Can you work these out from the model? Positions are in its coordinate system, mm. A direction names the side the tool comes from. Coordinates: 2 decimals unless noted, no trailing zeros. Order: outer loops, then holes, each group sorted by start corner. A loop starts at its lowest first (then second) coordinate and runs counter-clockwise, first axis right, second up. Notation, with made-up numbers: (-38.5, 0.5) -> (-8.5, 0.5) arc R35 cw to (-8.5, 36.5) -> close; hole circle Ø11 at (-13.5, -11.75). An arc over 180 degrees is marked (long way). Write item = value, one per line.
```python
from build123d import *
from OCP.BRepFilletAPI import BRepFilletAPI_MakeChamfer

# Parameters (mm, degrees)
SKETCH2_W           = 25.25
SKETCH2_H           = 38.25
SKETCH2_R           = 1.5
SKETCH2_W_2         = 19
SKETCH2_H_2         = 28.5
SKETCH2_R_2         = 1
BOSS_EXTRUDE1_DEPTH = 3
CHAMFER1_SIZE       = 0.5
CHAMFER1_SIZE2      = 0.360555128
CHAMFER1_SIZE2_2    = 0.382352941
CUT_EXTRUDE1_DEPTH  = 2
SKETCH5_R           = 1.5
SKETCH5_W           = 21
SKETCH5_H           = 28.5
BOSS_EXTRUDE2_DEPTH = 2.5


with BuildPart() as part:
    # Sketch2 → Boss-Extrude1 (new body)
    with BuildSketch(Plane.XY):
        Rectangle(SKETCH2_W, SKETCH2_H)
        with Locations((-10, -16.5)):
            Circle(SKETCH2_R, mode=Mode.SUBTRACT)
        with Locations((10, -16.5)):
            Circle(SKETCH2_R, mode=Mode.SUBTRACT)
        with Locations((10, 16.5)):
            Circle(SKETCH2_R, mode=Mode.SUBTRACT)
        with Locations((-10, 16.5)):
            Circle(SKETCH2_R, mode=Mode.SUBTRACT)
        Rectangle(SKETCH2_W_2, SKETCH2_H_2, mode=Mode.SUBTRACT)
        Polygon((-1.666666667, -1), (-1, 0), (-1.666666667, 1), (-9.5, 1), (-9.5, -1), align=None)
        with BuildLine():
            Line((-9.5, -14.25), (-8.833333333, -14.25))
            Line((-8.833333333, -14.25), (0, -1))
            ThreePointArc((0, -1), (-0.707106781, -0.707106781), (-1, 0))
            Line((-1, 0), (-1.666666667, -1))
            Line((-1.666666667, -1), (-9.5, -12.75))
            Line((-9.5, -12.75), (-9.5, -14.25))
        make_face()
        with BuildLine():
            Line((8.833333333, -14.25), (9.5, -14.25))
            Line((9.5, -14.25), (9.5, -12.75))
            Line((9.5, -12.75), (1.666666667, -1))
            Line((1.666666667, -1), (1, 0))
            ThreePointArc((1, 0), (0.707106781, -0.707106781), (0, -1))
            Line((0, -1), (8.833333333, -14.25))
        make_face()
        Polygon((1.666666667, -1), (9.5, -1), (9.5, 1), (1.666666667, 1), (1, 0), align=None)
        with BuildLine():
            ThreePointArc((0, 1), (0.707106781, 0.707106781), (1, 0))
            Line((1, 0), (1.666666667, 1))
            Line((1.666666667, 1), (9.5, 12.75))
            Line((9.5, 12.75), (9.5, 14.25))
            Line((9.5, 14.25), (8.833333333, 14.25))
            Line((8.833333333, 14.25), (0, 1))
        make_face()
        Circle(SKETCH2_R_2)
        with BuildLine():
            Line((-1.666666667, 1), (-1, 0))
            ThreePointArc((-1, 0), (-0.707106781, 0.707106781), (0, 1))
            Line((0, 1), (-8.833333333, 14.25))
            Line((-8.833333333, 14.25), (-9.5, 14.25))
            Line((-9.5, 14.25), (-9.5, 12.75))
            Line((-9.5, 12.75), (-1.666666667, 1))
        make_face()
    extrude(amount=BOSS_EXTRUDE1_DEPTH)

    # Chamfer1: one chamfer whose edges measure the first distance from different faces: ONE call of the kernel's chamfer builder (chamfer() names one face for all edges)
    chamfer1_edges_1 = [part.edges().sort_by_distance(p)[0] for p in [
        (-12.625, 19.125, 1.5),
        (12.625, 19.125, 1.5),
        (12.625, -19.125, 1.5),
        (-12.625, -19.125, 1.5),
        (-9.5, 1, 1.5),
        (-9.5, -1, 1.5),
        (9.5, -1, 1.5),
        (9.5, 1, 1.5),
    ]]
    chamfer1_edges_2 = [part.edges().sort_by_distance(p)[0] for p in [
        (-1.666666667, 1, 1.5),
    ]]
    chamfer1_side_2 = [part.faces().sort_by_distance(p)[0] for p in [
        (-5.583333333, 6.875, 1.5),
    ]]
    chamfer1_edges_3 = [part.edges().sort_by_distance(p)[0] for p in [
        (-9.5, 12.75, 1.5),
    ]]
    chamfer1_side_3 = [part.faces().sort_by_distance(p)[0] for p in [
        (-9.5, 6.875, 1.5),
    ]]
    chamfer1_edges_4 = [part.edges().sort_by_distance(p)[0] for p in [
        (-1.666666667, -1, 1.5),
    ]]
    chamfer1_side_4 = [part.faces().sort_by_distance(p)[0] for p in [
        (-5.583333333, -1, 1.5),
    ]]
    chamfer1_edges_5 = [part.edges().sort_by_distance(p)[0] for p in [
        (-9.5, -12.75, 1.5),
    ]]
    chamfer1_side_5 = [part.faces().sort_by_distance(p)[0] for p in [
        (-5.583333333, -6.875, 1.5),
    ]]
    chamfer1_edges_6 = [part.edges().sort_by_distance(p)[0] for p in [
        (8.833333333, 14.25, 1.5),
    ]]
    chamfer1_side_6 = [part.faces().sort_by_distance(p)[0] for p in [
        (0, 14.25, 1.5),
    ]]
    chamfer1_edges_7 = [part.edges().sort_by_distance(p)[0] for p in [
        (-8.833333333, 14.25, 1.5),
    ]]
    chamfer1_side_7 = [part.faces().sort_by_distance(p)[0] for p in [
        (-4.416666667, 7.625, 1.5),
    ]]
    chamfer1_edges_8 = [part.edges().sort_by_distance(p)[0] for p in [
        (0, 1, 1.5),
    ]]
    chamfer1_side_8 = [part.faces().sort_by_distance(p)[0] for p in [
        (4.416666667, 7.625, 1.5),
    ]]
    chamfer1_edges_9 = [part.edges().sort_by_distance(p)[0] for p in [
        (9.5, -12.75, 1.5),
    ]]
    chamfer1_side_9 = [part.faces().sort_by_distance(p)[0] for p in [
        (9.5, -6.875, 1.5),
    ]]
    chamfer1_edges_10 = [part.edges().sort_by_distance(p)[0] for p in [
        (1.666666667, -1, 1.5),
    ]]
    chamfer1_side_10 = [part.faces().sort_by_distance(p)[0] for p in [
        (5.583333333, -6.875, 1.5),
    ]]
    chamfer1_edges_11 = [part.edges().sort_by_distance(p)[0] for p in [
        (-8.833333333, -14.25, 1.5),
    ]]
    chamfer1_side_11 = [part.faces().sort_by_distance(p)[0] for p in [
        (0, -14.25, 1.5),
    ]]
    chamfer1_edges_12 = [part.edges().sort_by_distance(p)[0] for p in [
        (8.833333333, -14.25, 1.5),
    ]]
    chamfer1_side_12 = [part.faces().sort_by_distance(p)[0] for p in [
        (4.416666667, -7.625, 1.5),
    ]]
    chamfer1_edges_13 = [part.edges().sort_by_distance(p)[0] for p in [
        (0, -1, 1.5),
    ]]
    chamfer1_side_13 = [part.faces().sort_by_distance(p)[0] for p in [
        (-4.416666667, -7.625, 1.5),
    ]]
    chamfer1_edges_14 = [part.edges().sort_by_distance(p)[0] for p in [
        (9.5, 12.75, 1.5),
    ]]
    chamfer1_side_14 = [part.faces().sort_by_distance(p)[0] for p in [
        (5.583333333, 6.875, 1.5),
    ]]
    chamfer1 = BRepFilletAPI_MakeChamfer(part.part.solid().wrapped)
    for e in chamfer1_edges_1:
        chamfer1.Add(CHAMFER1_SIZE, e.wrapped)
    for e in chamfer1_edges_2:
        chamfer1.Add(CHAMFER1_SIZE, CHAMFER1_SIZE2, e.wrapped, chamfer1_side_2[0].wrapped)  # the first distance lies on this face
    for e in chamfer1_edges_3:
        chamfer1.Add(CHAMFER1_SIZE, CHAMFER1_SIZE2, e.wrapped, chamfer1_side_3[0].wrapped)  # the first distance lies on this face
    for e in chamfer1_edges_4:
        chamfer1.Add(CHAMFER1_SIZE, CHAMFER1_SIZE2, e.wrapped, chamfer1_side_4[0].wrapped)  # the first distance lies on this face
    for e in chamfer1_edges_5:
        chamfer1.Add(CHAMFER1_SIZE, CHAMFER1_SIZE2, e.wrapped, chamfer1_side_5[0].wrapped)  # the first distance lies on this face
    for e in chamfer1_edges_6:
        chamfer1.Add(CHAMFER1_SIZE, CHAMFER1_SIZE2, e.wrapped, chamfer1_side_6[0].wrapped)  # the first distance lies on this face
    for e in chamfer1_edges_7:
        chamfer1.Add(CHAMFER1_SIZE, CHAMFER1_SIZE2, e.wrapped, chamfer1_side_7[0].wrapped)  # the first distance lies on this face
    for e in chamfer1_edges_8:
        chamfer1.Add(CHAMFER1_SIZE, CHAMFER1_SIZE2_2, e.wrapped, chamfer1_side_8[0].wrapped)  # the first distance lies on this face
    for e in chamfer1_edges_9:
        chamfer1.Add(CHAMFER1_SIZE, CHAMFER1_SIZE2, e.wrapped, chamfer1_side_9[0].wrapped)  # the first distance lies on this face
    for e in chamfer1_edges_10:
        chamfer1.Add(CHAMFER1_SIZE, CHAMFER1_SIZE2, e.wrapped, chamfer1_side_10[0].wrapped)  # the first distance lies on this face
    for e in chamfer1_edges_11:
        chamfer1.Add(CHAMFER1_SIZE, CHAMFER1_SIZE2, e.wrapped, chamfer1_side_11[0].wrapped)  # the first distance lies on this face
    for e in chamfer1_edges_12:
        chamfer1.Add(CHAMFER1_SIZE, CHAMFER1_SIZE2, e.wrapped, chamfer1_side_12[0].wrapped)  # the first distance lies on this face
    for e in chamfer1_edges_13:
        chamfer1.Add(CHAMFER1_SIZE, CHAMFER1_SIZE2_2, e.wrapped, chamfer1_side_13[0].wrapped)  # the first distance lies on this face
    for e in chamfer1_edges_14:
        chamfer1.Add(CHAMFER1_SIZE, CHAMFER1_SIZE2, e.wrapped, chamfer1_side_14[0].wrapped)  # the first distance lies on this face
    add(Compound.cast(chamfer1.Shape()), mode=Mode.REPLACE)

    # Sketch3 → Cut-Extrude1 (cut)
    with BuildSketch(Plane(origin=(0, 0, 0), x_dir=(-1, 0, 0), z_dir=(0, 0, -1))):
        Polygon((10.5, -14.25), (10.5, 14.25), (8.472778206, 14.25), (8.555983235, 13.833974853), (0.212091251, 1.318136877), (-0.277350098, 1.416025147), (-8.633333333, 13.95), (-8.333333333, 14.25), (-10.5, 14.25), (-10.5, -14.25), (-8.472778206, -14.25), (-8.555983235, -13.833974853), (-0.212091251, -1.318136877), (0.277350098, -1.416025147), (8.633333333, -13.95), (8.333333333, -14.25), align=None)
        Polygon((-1.666666667, 1), (-9, 1), (-9.5, 1.5), (-9.5, 12.389444872), (-9.222649902, 12.333974853), align=None, mode=Mode.SUBTRACT)
        Polygon((-9.5, -1.5), (-9, -1), (-2.027221794, -1), (-1.944016765, -1.416025147), (-9.3, -12.45), (-9.5, -12.25), align=None, mode=Mode.SUBTRACT)
        Polygon((9.5, 1.5), (9, 1), (2.027221794, 1), (1.944016765, 1.416025147), (9.3, 12.45), (9.5, 12.25), align=None, mode=Mode.SUBTRACT)
        Polygon((9.222649902, -12.333974853), (1.866666667, -1.3), (2.166666667, -1), (9, -1), (9.5, -1.5), (9.5, -12.389444872), align=None, mode=Mode.SUBTRACT)
    extrude(amount=-CUT_EXTRUDE1_DEPTH, mode=Mode.SUBTRACT)

    # Sketch5 → Boss-Extrude2 (add)
    with BuildSketch(Plane(origin=(0, 0, 0), x_dir=(-1, 0, 0), z_dir=(0, 0, -1))):
        Polygon((-12.125, -19.125), (12.125, -19.125), (12.625, -18.625), (12.625, 18.625), (12.125, 19.125), (-12.125, 19.125), (-12.625, 18.625), (-12.625, -18.625), align=None)
        with Locations((-10, -16.5)):
            Circle(SKETCH5_R, mode=Mode.SUBTRACT)
        with Locations((10, -16.5)):
            Circle(SKETCH5_R, mode=Mode.SUBTRACT)
        with Locations((10, 16.5)):
            Circle(SKETCH5_R, mode=Mode.SUBTRACT)
        with Locations((-10, 16.5)):
            Circle(SKETCH5_R, mode=Mode.SUBTRACT)
        Rectangle(SKETCH5_W, SKETCH5_H, mode=Mode.SUBTRACT)
    extrude(amount=BOSS_EXTRUDE2_DEPTH)


solid = part.part
```
Item 1: If I drill on probe 1 along X at (y, z) = (-16.5, 1.2) (3 decimals); probe 2 along Y at (x, z) = (10, -0.6) (3 decimals); probe 3 along Y at (x, z) = (10, 2.05) (3 decimals), over which ranges is the centre line in solid material (lowest first)?
A:
probe_1 = -12.625 to -11.5, -8.5 to 8.5, 11.5 to 12.625
probe_2 = -19.125 to -18, -15 to -14.25, 14.25 to 15, 18 to 19.125
probe_3 = -19.125 to -18, -15 to 15, 18 to 19.125
Item 2: I want a section at B-B, the plane x = 3. Please give me the cut outline in (y, z) (3 decimals), plus the area to 3 significant figures.
A:
outline = (-19.125, -2.5) -> (-14.25, -2.5) -> (-14.25, 3) -> (-19.125, 3) -> close; (-5.5, 2) -> (-3, 2) -> (-3, 3) -> (-5.5, 3) -> close; (-1, 2) -> (1, 2) -> (1, 3) -> (-1, 3) -> close; (3, 2) -> (5.5, 2) -> (5.5, 3) -> (3, 3) -> close; (14.25, -2.5) -> (19.125, -2.5) -> (19.125, 3) -> (14.25, 3) -> close
area = 60.6 mm2
Item 3: I want a section at C-C, the plane x = 10. Please give me the cut outline in (y, z) (3 decimals), plus the area to 3 significant figures.
A:
outline = (-19.125, -2.5) -> (-18, -2.5) -> (-18, 3) -> (-19.125, 3) -> close; (-15, -2.5) -> (-14.25, -2.5) -> (-14.25, 2) -> (14.25, 2) -> (14.25, -2.5) -> (15, -2.5) -> (15, 3) -> (-15, 3) -> close; (18, -2.5) -> (19.125, -2.5) -> (19.125, 3) -> (18, 3) -> close
area = 49.1 mm2
Item 4: I want a section at D-D, the plane z = -1.85. Please give me the cut outline in (x, y) (3 decimals), plus the area to 3 significant figures.
A:
outline = (-12.625, -18.625) -> (-12.125, -19.125) -> (12.125, -19.125) -> (12.625, -18.625) -> (12.625, 18.625) -> (12.125, 19.125) -> (-12.125, 19.125) -> (-12.625, 18.625) -> close; hole circle Ø3 at (-10, -16.5); hole circle Ø3 at (-10, 16.5); hole (-10.5, -14.25) -> (10.5, -14.25) -> (10.5, 14.25) -> (-10.5, 14.25) -> close; hole circle Ø3 at (10, -16.5); hole circle Ø3 at (10, 16.5)
area = 339 mm2
Item 5: I want a section at A-A, the plane y = -13. Please give me the cut outline in (x, z) (3 decimals).
A:
outline = (-12.625, -2.5) -> (-10.5, -2.5) -> (-10.5, 2) -> (-8, 2) -> (-8, 3) -> (-12.625, 3) -> close; (8, 2) -> (10.5, 2) -> (10.5, -2.5) -> (12.625, -2.5) -> (12.625, 3) -> (8, 3) -> close
Item 6: I'm going to push a flat-ended pin straight in: P1, Ø8, axis at x = -5, y = 9.5, coming from the -Z side. Where does the tip first touch, or does it pass through?
A:
P1 = 2
Item 7: If we mould it in two halves opening along Y, with no side actions, what happens to faces 1 (the flat face through (0, 19.125, 0)), 2 (the flat face through (-12.625, 0, 0)), 3 (the flat face through (-5.6, -1, 2.5))? For each: pulls with the +Y half, pulls with the -Y half, needs draft (parallel to the pull), parting line crosses it, or undercut.
A:
face_1 = pulls with the +Y half
face_2 = needs draft
face_3 = undercut
Item 8: For faces 4 (the flat face through (9.5, -7, 2.5)), 5 (the flat face through (0, 0, 2)), 6 (the flat face through (12.625, 0, 0)), which set-ups out of +Z, -Z, +X, -X, +Y, -Y let a thin tool reach every point of the face, with its end or its side?
A:
face_4 = +Z, -Z
face_5 = -Z
face_6 = +Z, -Z, +X, +Y, -Y
